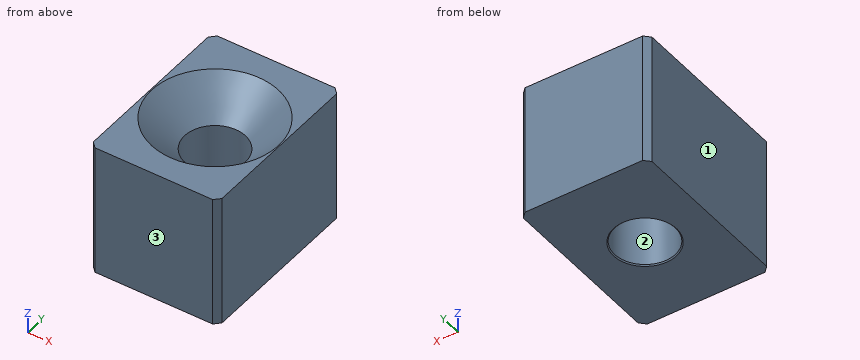
Autodesk Inventor part; units mm, degrees
ref_plane "YZ Plane" through (0, 0, 0) normal (1, 0, 0) x (0, 1, 0)
ref_plane "XZ Plane" through (0, 0, 0) normal (0, 1, 0) x (-1, 0, 0)
ref_plane "XY Plane" through (0, 0, 0) normal (0, 0, 1) x (1, 0, 0)
sketch "Sketch1" plane through (0, 0, 0) normal (0, 0, 1) x (1, 0, 0)
  line L0 (23.825, 8.05) -> (23.825, -8.05) construction
  line L1 (37, 8) -> (31.3548, 8) construction
  line L2 (31.3548, -8) -> (37, -8) construction
  line L3 (37, 8) -> (23.825, 8) construction
  line L4 (23.825, 8) -> (23.825, -8) construction
  line L5 (23.825, -8) -> (37, -8) construction
  line L6 (37, -8) -> (37, 8) construction
  circle A0 centre (30.6625, 0) radius 2.067 construction
  line L7 (36.5, -8) -> (24.825, -8)
  line L8 (24.825, -8) -> (24.825, 8)
  line L9 (24.825, 8) -> (36.5, 8)
  line L10 (36.5, 8) -> (36.5, -8)
  line L11 (36.5, -8) -> (24.825, 8) construction
  line L12 (24.825, -8) -> (36.5, 8) construction
  point P0 (0, 0)
  dimension "d0" = 1
  dimension "d1" = 0
  dimension "d11" = 11.675
  dimension "d12" = 16
extrude "Extrusion1" add sketch "Sketch1" along normal blind 12
sketch "Sketch2" plane through (0, 0, 12) normal (0, 0, 1) x (1, 0, 0)
  point P0 (0, 0)
  point P1 (30.6625, 0)
hole "Hole1" at (30.6625, 0, 12) direction (0, 0, -1) diameter 5.5 end through all countersink diameter 11.5 countersink angle 90
chamfer "Chamfer1" distance 0.5 angle 45 4 edges at (24.825, -8, 6) (24.825, 8, 6) (36.5, 8, 6) (36.5, -8, 6)
chamfer "Chamfer2" distance 0.1 angle 45 1 edges at (30.6625, 2.75, 0)
properties part number "TH1-002" material "Steel, Mild"
Verification items for the finished model (mm, model axes). Face numbers are marked on the shaded views. Coordinates: 2 decimals unless noted, no trailing zeros. Answer as a JSON object with one key per item and string values.
(1) Gauge pin test, flat ends, axial feed: pin 1 Ø1.5 at (x, y) = (32, -3.5) entering from +Z; pin 2 Ø3 at (x, y) = (30, 4) entering from +Z. Record the tip position at first contact, or that the pin passes through.
Report:
{"pin 1": "z = 10.75", "pin 2": "z = 11.8"}
(2) Mould release check, pull along X, two halves, no side actions. Record for the marked faces 1, 2 and 3: pulls with the +X half, pulls with the -X half, needs draft (parallel to the pull), parting line crosses it, or undercut.
Report:
{"face 1": "pulls with the -X half", "face 2": "undercut", "face 3": "needs draft"}
(3) Thickness scan on line 1 along X through (y, z) = (0, 2) (1 decimal); line 2 along Y through (x, z) = (27.75, 10.5); line 3 along X through (y, z) = (-0.75, 4) (3 decimals). Record the ranges inside material, lowest first.
Report:
{"line 1": "24.8 to 27.9, 33.4 to 36.5", "line 2": "-8 to -3.1, 3.1 to 8", "line 3": "24.825 to 28.017, 33.308 to 36.5"}
